Check sheet for the modelled part. Datum: model origin and axes. Units: mm. A direction names the side the tool comes from. Round coordinates to 2 decimals unless told otherwise and drop trailing zeros. Write each loop counter-clockwise with the first axis right and the second up, starting at its lowest first coordinate (ties: lowest second). Pieces come first, ordered by that corner, then holes. Notation, with made-up numbers: (63.25, 79) - (115.25, 79) arc R25 cw to (115.25, 91) - close; hole circle Ø11 at (52.25, -29). An arc over 180 degrees is marked (long way). Answer as a JSON object with one key per item and string values. Group by question number.
Item 1: Sectioned sample at D-D on y = 2.75. Record the boundary of the cut face in (x, z).
Item 2: Release check for a two-part mould opening along Y. For faces 1 (the flat face through (2, -6.35, 9)), 2 (the flat face through (0, 0, 12.7)), 3 (the cylindrical face through (-0.69, -3.1, 6.26)), 4 (the cylindrical face through (-0.41, 7.92, 9.37)) record: pulls with the +Y half, pulls with the -Y half, needs draft (parallel to the pull), parting line crosses it, or undercut.
Item 3: Sectioned sample at B-B on y = 0. Record the boundary of the cut face in (x, z) (3 decimals).
Item 4: Sectioned sample at C-C on y = 5. Record the boundary of the cut face in (x, z).
Item 5: Thickness scan on line 1 (Y direction, x = 0, z = 7.5) (3 decimals); line 2 (Y direction, x = 0, z = 10) (3 decimals); line 3 (X direction, y = -2.75, z = 10.25). Record the ranges inside material, lowest first.
Item 6: Gauge pin test, flat ends, axial feed: P1, Ø3, axis at x = -3, y = 1, coming from the +Z side; P2, Ø10, axis at x = 0, y = 0, coming from the -Z side; P3, Ø3, axis at x = 1, y = 0.5, coming from the -Z side; P4, Ø1, axis at y = 7, z = 12.5, coming from the +X side. Record the tip position at first contact, or that the pin passes through.
Item 7: Set-up check for faces 5 (the cylindrical face through (-0.41, -7.83, 9.37)), 6 (the cylindrical face through (0.33, -0.09, 17.14)): record each of +Z, -Z, +X, -X, +Y, -Y from which the full face is reachable in a straight line by a thin tool's end or side.
Item 8: Sectioned sample at A-A on x = 0. Record the boundary of the cut face in (y, z) (3 decimals).
```python
from build123d import *

# Parameters (mm, degrees)
F3_DEPTH = 6.35
F1_R     = 3.175
F4_DEPTH = 9.525
F2_R     = 3.175
F5_DEPTH = 12.7
F6_R     = 0.254


with BuildPart() as f3:
    # F0 (on Front) → F3 (new body, symmetric)
    with BuildSketch(Plane.XZ):
        with BuildLine():
            Line((-8.9757648699, 0), (8.9757648699, 0))
            ThreePointArc((8.9757648699, 0), (0, 17.145), (-8.9757648699, 0))
        make_face()
    extrude(amount=F3_DEPTH, both=True)

    # F1 (on Front) → F4 (join, symmetric)
    with BuildSketch(Plane.XZ):
        with Locations((0, 6.223)):
            Circle(F1_R)
    extrude(amount=F4_DEPTH, both=True)

    # F2 (on Top) → F5 (cut)
    with BuildSketch(Plane.XY):
        Circle(F2_R)
    extrude(amount=F5_DEPTH, mode=Mode.SUBTRACT)

    # F6
    f6_edges = [f3.edges().sort_by_distance(p)[0] for p in [
        (0, -6.35, 17.145),
        (0, 6.35, 17.145),
        (8.975765, 0, 0),
        (0, -6.35, 0),
        (-3.175, -9.525, 6.223),
        (0, 6.35, 0),
        (-8.975765, 0, 0),
    ]]
    fillet(f6_edges, radius=F6_R)


solid = f3.part
```
Completed:
{
 "1": {"outline": "(-9.05, 0.11) arc R0.25 ccw to (-8.84, 0) - (-1.59, 0) - (-1.59, 12.7) - (1.59, 12.7) - (1.59, 0) - (8.84, 0) arc R0.25 ccw to (9.05, 0.11) arc R10.92 ccw (long way) to start"},
 "2": {"face 1": "pulls with the -Y half", "face 2": "undercut", "face 3": "undercut", "face 4": "needs draft"},
 "3": {"outline": "(-9.052, 0.112) arc R0.254 ccw to (-8.842, 0) - (-3.175, 0) - (-3.175, 12.7) - (3.175, 12.7) - (3.175, 0) - (8.842, 0) arc R0.254 ccw to (9.052, 0.112) arc R10.922 ccw (long way) to start"},
 "4": {"outline": "(-9.05, 0.11) arc R0.25 ccw to (-8.84, 0) - (8.84, 0) arc R0.25 ccw to (9.05, 0.11) arc R10.92 ccw (long way) to start"},
 "5": {"line 1": "-9.525 to -3.175, 3.175 to 9.525", "line 2": "-6.35 to -3.175, 3.175 to 6.35", "line 3": "-10.15 to -1.59, 1.59 to 10.15"},
 "6": {"P1": "z = 17.04", "P2": "z = 0", "P3": "z = 12.7", "P4": "through"},
 "7": {"face 5": "-Y", "face 6": "+Y, -Y"},
 "8": {"outline": "(-9.525, 3.302) arc R0.254 ccw to (-9.271, 3.048) - (-6.35, 3.048) - (-6.35, 0.254) arc R0.254 ccw to (-6.096, 0) - (-3.175, 0) - (-3.175, 12.7) - (3.175, 12.7) - (3.175, 0) - (6.096, 0) arc R0.254 ccw to (6.35, 0.254) - (6.35, 3.048) - (9.525, 3.048) - (9.525, 9.398) - (6.35, 9.398) - (6.35, 16.891) arc R0.254 ccw to (6.096, 17.145) - (-6.096, 17.145) arc R0.254 ccw to (-6.35, 16.891) - (-6.35, 9.398) - (-9.271, 9.398) arc R0.254 ccw to (-9.525, 9.144) - close"}
}
